Build history of the part. All positions in model axes, mm. Face numbers are marked on the shaded views. A direction names the side the tool comes from. Give positions to 0.01 mm unless a question says otherwise; leave off trailing zeros. Use a Markdown table: item, result.
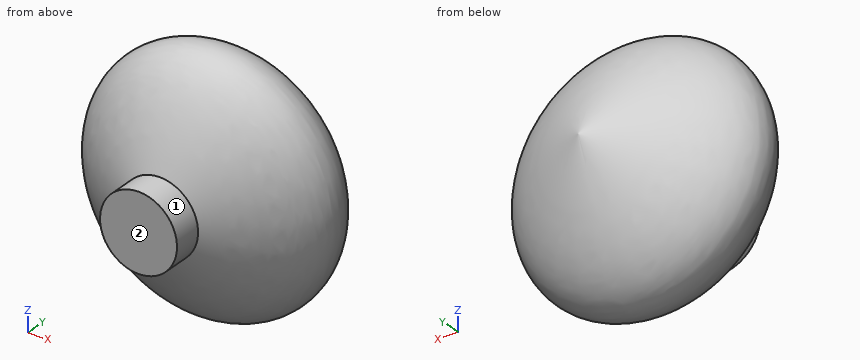
from build123d import *

# Parameters (mm, degrees)
SKETCH9_R           = 2
BOSS_EXTRUDE1_DEPTH = 2


with BuildPart() as part:
    # Sketch5 → Revolve2 (revolve)
    with BuildSketch(Plane(origin=(0, 0, 0), x_dir=(0, 0, -1), z_dir=(1, 0, 0))):
        with BuildLine():
            Line((0, -1.305492492), (0, 8.226206899))
            add(Edge.make_bspline(
                [(0, 8.226206899), (12.899965566, 3.460357203), (0, -1.305492492)],
                knots=[0, 0, 0, 1, 1, 1], degree=2))
        make_face()
    revolve(axis=Axis((0, -1.305492492, 0), (0, 1, 0)))

    # Sketch9 → Boss-Extrude1 (add)
    with BuildSketch(Plane(origin=(0, 0, 0), x_dir=(1, 0, 0), z_dir=(0, 1, 0))):
        with Locations(Location((0, 0, 0), (0, 0, 270))):
            Circle(SKETCH9_R)
    extrude(amount=-BOSS_EXTRUDE1_DEPTH)


solid = part.part
1) Tool access for the marked faces 1 and 2: list every direction of +Z, -Z, +X, -X, +Y, -Y with a clear straight run to the whole face (end or side of a thin tool).
Computed:
| item | result |
|---|---|
| face 1 | -Y |
| face 2 | +Z, -Z, +X, -X, -Y |
2) Wall check: line 1 (Z direction, x = 0, y = -1); line 2 (X direction, y = 2.5, z = 3.5); line 3 (Y direction, x = 3.5, z = -4.75). Give the ranges that are in metal, low to high. Write a range as from..to.
Computed:
| item | result |
|---|---|
| line 1 | z = -2..2 |
| line 2 | x = -5.1..5.1 |
| line 3 | y = 2.07..4.85 |
3) Pin check, flat tips, straight feed: P1, Ø1.5, axis at x = 2, z = 1.5, coming from the -Y side; P2, Ø6, axis at x = 2, y = 7, coming from the -Z side; P3, Ø4, axis at x = -0.5, y = 6.5, coming from the +Z side; P4, Ø1.5, axis at x = -1, z = 4.5, coming from the -Y side. Stop position of each tip, or through.
Computed:
| item | result |
|---|---|
| P1 | stops at y = -2 |
| P2 | stops at z = -6.23 |
| P3 | stops at z = 6.13 |
| P4 | stops at y = 0.44 |
